Here's how the part is built. I have some questions about the finished solid (model axes, mm). Coordinates: 2 decimals unless noted, no trailing zeros. Order: outer loops, then holes, each group sorted by start corner. A loop starts at its lowest first (then second) coordinate and runs counter-clockwise, first axis right, second up. Notation, with made-up numbers: (48, 85) - (87, 85) arc R13 cw to (87, 96) - close; hole circle Ø8 at (-17, 70). An arc over 180 degrees is marked (long way). Answer in a Markdown table with one row per item. Add a question column.
Item 1: I want a section at D-D (z = -186.5). Please give me the cut outline in (x, y).
Item 2: I want a section at C-C (y = 1.5). Count the separate pieces of the cut face and the enclosed holes in it, plus the area to 3 significant figures.
Item 3: I want a section at B-B (z = -217). Please give me the cut outline in (x, y), plus the area to 3 significant figures.
Item 4: If I drill on line 1 along Z through (x, y) = (130, 1.65); line 2 along Z through (x, y) = (59, 1.75); line 3 along Z through (x, y) = (102, 2.3), over which ranges is the centre line in solid material (lowest first)? Write a range as from..to.
Item 5: I want a section at A-A (x = 86). Please give me the cut outline in (y, z).
Autodesk Inventor part; units mm, degrees
ref_plane "YZ Plane" through (0, 0, 0) normal (1, 0, 0) x (0, 1, 0)
ref_plane "XZ Plane" through (0, 0, 0) normal (0, 1, 0) x (-1, 0, 0)
ref_plane "XY Plane" through (0, 0, 0) normal (0, 0, 1) x (1, 0, 0)
sketch "Sketch1" plane through (0, 0, 0) normal (0, 1, 0) x (-1, 0, 0)
  circle A0 centre (0, 0) radius 215
  circle A1 centre (0, 0) radius 315
  line L0 (0, 0) -> (0, -315)
  line L1 (0, 0) -> (-222.7386, -222.7386)
  line L2 (-141.0509, -162.2641) -> (-211.8794, -233.0926)
  line L3 (-15, -214.4761) -> (-15, -314.6427)
  circle A2 centre (0, 0) radius 222.5
  circle A3 centre (0, 0) radius 307.5
  line L4 (-18, -214.2452) -> (-18, -314.4853)
  point P0 (-152.028, -152.028)
  point P1 (0, -215)
  point P2 (0, -312.5)
  point P3 (0, -217.5)
  point P4 (-153.7957, -153.7957)
  point P5 (-220.9709, -220.9709)
  point P6 (-210.1096, -231.3228)
  point P7 (-15, -312.1398)
  point P8 (-15, -216.9821)
  point P9 (-142.8229, -164.0361)
  point P10 (-206.5699, -227.7831)
  point P11 (-15, -307.1339)
  point P12 (-15, -221.9938)
  point P13 (-146.3667, -167.5799)
  point P14 (-18, -306.9727)
  point P15 (-18, -221.7707)
  dimension "d2" = 430
  dimension "d3" = 630
  dimension "d4" = 45
  dimension "d5" = 15
  dimension "d6" = 15
  dimension "d11" = 7.5
  dimension "d12" = 7.5
  dimension "d13" = 3
extrude "Extrusion1" add sketch "Sketch1" along normal blind 3 contours A2 L4 A3 L2
sketch "Sketch5" plane through (0, 3, 0) normal (0, 1, 0) x (1, 0, 0)
  arc A0 (146.3667, 167.5799) -> (18, 221.7707) centre (0, 0) ccw
  line L0 (146.3667, 167.5799) -> (206.5699, 227.7831)
  arc A1 (206.5699, 227.7831) -> (18, 306.9727) centre (0, 0) ccw
  line L1 (18, 306.9727) -> (18, 221.7707)
  circle A2 centre (0, 0) radius 297.5
  circle A3 centre (0, 0) radius 232.5
  line L2 (28, 296.1794) -> (28, 230.8078)
  line L3 (145.7715, 181.1268) -> (191.9425, 227.2979)
  line L4 (18, 306.9727) -> (18, 221.7707)
  line L5 (18, 296.955) -> (18, 231.8022)
  line L6 (146.3667, 167.5799) -> (206.5699, 227.7831)
  line L7 (199.4901, 220.7033) -> (153.4532, 174.6664)
  dimension "d43" = 10
  dimension "d44" = 10
  dimension "d45" = 10
  dimension "d46" = 10
sketch "Sketch6" plane through (0, 3, 0) normal (0, 1, 0) x (1, 0, 0)
  arc A0 (146.3667, 167.5799) -> (18, 221.7707) centre (0, 0) ccw
  line L0 (146.3667, 167.5799) -> (206.5699, 227.7831)
  arc A1 (206.5699, 227.7831) -> (18, 306.9727) centre (0, 0) ccw
  line L1 (18, 306.9727) -> (18, 221.7707)
  circle A2 centre (0, 0) radius 222.5
  circle A3 centre (0, 0) radius 309.5
  circle A4 centre (0, 0) radius 240
  circle A5 centre (0, 0) radius 290
  line L2 (18, 306.9727) -> (18, 221.7707)
  line L3 (18, 239.324) -> (18, 289.4408)
  line L4 (146.3667, 167.5799) -> (206.5699, 227.7831)
  line L5 (158.7672, 179.9804) -> (194.1799, 215.3931)
  line L6 (50, 234.7339) -> (50, 285.6571)
  line L7 (130.6266, 201.3373) -> (166.6348, 237.3454)
  line L8 (55, 233.6129) -> (55, 284.7367)
  line L9 (126.2984, 204.0802) -> (162.4484, 240.2301)
  circle A6 centre (0, 0) radius 245
  circle A7 centre (0, 0) radius 285
  line L10 (55, 274.8261) -> (59, 274.8261) construction
  line L11 (59, 274.8261) -> (59, 278.8261) construction
  line L12 (55, 241.7898) -> (59, 241.7898) construction
  line L13 (59, 241.7898) -> (59, 237.7898) construction
  line L14 (132.0804, 209.8621) -> (129.2519, 212.6905) construction
  line L15 (129.2519, 212.6905) -> (126.4235, 209.8621) construction
  line L16 (155.4405, 233.2223) -> (152.6121, 236.0507) construction
  line L17 (152.6121, 236.0507) -> (155.4405, 238.8791) construction
  circle A8 centre (152.6121, 236.0507) radius 1.75
  circle A9 centre (129.2519, 212.6905) radius 1.75
  circle A10 centre (59, 274.8261) radius 1.75
  circle A11 centre (59, 241.7898) radius 1.75
  line L18 (15, 221.9938) -> (15, 309.1363)
  line L19 (0, 449.6314) -> (0, -436.0219)
  point P0 (176.4736, 197.6868)
  dimension "d47" = 445
  dimension "d48" = 619
  dimension "d49" = 480
  dimension "d50" = 580
  dimension "d53" = 5
  dimension "d54" = 5
  dimension "d55" = 5
  dimension "d56" = 5
  dimension "d57" = 4
  dimension "d58" = 4
  dimension "d59" = 4
  dimension "d60" = 4
  dimension "d61" = 4
  dimension "d63" = 4
  dimension "d67" = 90
  dimension "d68" = 4
  dimension "d69" = 4
  dimension "d70" = 3.5
  dimension "d71" = 3.5
  dimension "d72" = 3.5
  dimension "d73" = 3.5
  dimension "d76" = 35
  dimension "d77" = 15
  dimension "d78" = 35
extrude "Extrusion4" cut sketch "Sketch6" against normal up to next contours A8 | A9 | A10 | A11
sketch "Sketch8" plane through (0, 3, 0) normal (0, 1, 0) x (1, 0, 0)
  circle A0 centre (129.2519, 212.6905) radius 1.75
  circle A1 centre (59, 274.8261) radius 1.75
  circle A2 centre (152.6121, 236.0507) radius 1.75
  circle A3 centre (59, 241.7898) radius 1.75
  arc A4 (146.3667, 167.5799) -> (18, 221.7707) centre (0, 0) ccw
  line L0 (146.3667, 167.5799) -> (206.5699, 227.7831)
  arc A5 (206.5699, 227.7831) -> (18, 306.9727) centre (0, 0) ccw
  line L1 (18, 306.9727) -> (18, 221.7707)
  circle A6 centre (129.2519, 212.6905) radius 1.75
  circle A7 centre (59, 241.7898) radius 1.75
  circle A8 centre (152.6121, 236.0507) radius 1.75
  circle A9 centre (0, 0) radius 248.8841 construction
  circle A10 centre (59, 274.8261) radius 1.75
  circle A11 centre (0, 0) radius 281.0879 construction
  circle A12 centre (0, 0) radius 245.8841
  circle A13 centre (0, 0) radius 284.0879
  line L2 (59, 241.7898) -> (59, 274.8261) construction
  line L3 (129.2519, 212.6905) -> (152.6121, 236.0507) construction
  line L4 (122.6187, 213.1283) -> (150.4617, 240.9714)
  line L5 (64, 237.409) -> (64, 276.785)
  dimension "d96" = 3
  dimension "d97" = 3
  dimension "d98" = 5
  dimension "d100" = 5
extrude "Extrusion5" cut sketch "Sketch8" against normal up to next contours A0 | A1 | A2 | A3 | A12 L5 A13 L4
properties part number "Battery Module Third Iteration" material "PLA Plastic"
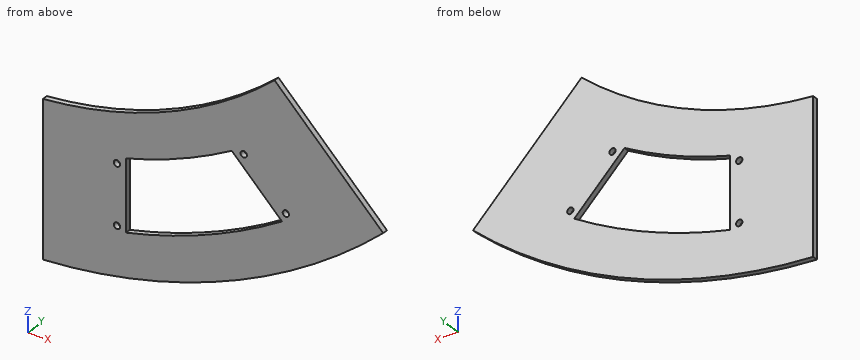
Values follow:
| question | item | result |
|---|---|---|
| 1 | outline | (121.34, 0) - (165.29, 0) - (165.29, 3) - (121.34, 3) - close |
| 2 | separate pieces | 1 |
| 2 | enclosed holes | 5 |
| 2 | area | 11,800 mm^2 |
| 3 | outline | (49.17, 0) - (115.63, 0) - (115.63, 3) - (49.17, 3) - close; (126.49, 0) - (195.79, 0) - (195.79, 3) - (126.49, 3) - close |
| 3 | area | 407 mm^2 |
| 4 | line 1 | z = -278.67..-252.6, -220.51..-214.27, -211.11..-180.57 |
| 4 | line 2 | z = -301.79..-276.58, -273.08..-243.54, -240.04..-214.53 |
| 4 | line 3 | z = -290.09..-265.15, -223.73..-197.74 |
| 5 | outline | (0, -295.23) - (3, -295.23) - (3, -270.76) - (0, -270.76) - close; (0, -230.35) - (3, -230.35) - (3, -205.21) - (0, -205.21) - close |
